from build123d import *

# Parameters (mm, degrees)
BOSS_EXTRUDE1_DEPTH   = 1.6
F_4_0MM_DOWEL_HOLE1_D = 4


with BuildPart() as part:
    # Sketch1 → Boss-Extrude1 (new body)
    with BuildSketch(Plane(origin=(0, 0, 0), x_dir=(1, 0, 0), z_dir=(0, 1, 0))):
        with BuildLine():
            ThreePointArc((-65, 33.226495452), (-73, 0), (-65, -33.226495452))
            ThreePointArc((-65, -33.226495452), (-51.618795027, -51.618795027), (-33.226495452, -65))
            ThreePointArc((-33.226495452, -65), (0, -73), (33.226495452, -65))
            ThreePointArc((33.226495452, -65), (51.618795027, -51.618795027), (65, -33.226495452))
            ThreePointArc((65, -33.226495452), (70.971825396, -17.088007491), (73, 0))
            ThreePointArc((73, 0), (70.971825396, 17.088007491), (65, 33.226495452))
            ThreePointArc((65, 33.226495452), (51.618795027, 51.618795027), (33.226495452, 65))
            ThreePointArc((33.226495452, 65), (0, 73), (-33.226495452, 65))
            ThreePointArc((-33.226495452, 65), (-51.618795027, 51.618795027), (-65, 33.226495452))
        make_face()
    extrude(amount=BOSS_EXTRUDE1_DEPTH)

    # Ø4.0mm Dowel Hole1 (through all)
    with Locations(Plane(origin=(0, 1.6, 0), x_dir=(1, 0, 0), z_dir=(0, 1, 0))):
        with Locations((0, 55), (55, 0), (-55, 0), (0, -55)):
            Hole(F_4_0MM_DOWEL_HOLE1_D / 2)


solid = part.part
Could you check a few things on this model? Use its own coordinates, in mm. Coordinates: 2 decimals unless noted, no trailing zeros. Order: outer loops, then holes, each group sorted by start corner. A loop starts at its lowest first (then second) coordinate and runs counter-clockwise, first axis right, second up. Notation, with made-up numbers: (46, -6) -> (86, -6) arc R23 cw to (86, 28) -> close; hole circle Ø6 at (-26.5, 38). An arc over 180 degrees is marked (long way). One line per item, written item: value. Start each with the question number.
1) Imagine slicing it at D-D on y = 0.8. List the corners of the cut face in (x, z) for me.
2) Imagine slicing it at A-A on x = 0. List the corners of the cut face in (y, z) for me.
3) Imagine slicing it at C-C on x = -55. List the corners of the cut face in (y, z) for me.
4) Imagine slicing it at B-B on z = 55. List the corners of the cut face in (x, y) for me, plus the area to 3 significant figures.
5) We'd pull the mould along X, two halves only. Please class faces 1 (the cylindrical face through (0, 1, 53)), 2 (the flat face through (-1, 0, -1)): +X half, -X half, draft (parallel to the pull), parting line (faces both ways), or undercut.
6) If I drill on L1, parallel to Z at x = 55, y = 0.6; L2, parallel to X at y = 0.3, z = -34.5, over which ranges is the centre line in solid material (lowest first)? Write a range as [from, to].
Answer list:
1. outline: circle Ø146 at (0, 0); hole circle Ø4 at (-55, 0); hole circle Ø4 at (0, -55); hole circle Ø4 at (0, 55); hole circle Ø4 at (55, 0)
2. outline: (0, -73) -> (1.6, -73) -> (1.6, -57) -> (0, -57) -> close; (0, -53) -> (1.6, -53) -> (1.6, 53) -> (0, 53) -> close; (0, 57) -> (1.6, 57) -> (1.6, 73) -> (0, 73) -> close
3. outline: (0, -48) -> (1.6, -48) -> (1.6, -2) -> (0, -2) -> close; (0, 2) -> (1.6, 2) -> (1.6, 48) -> (0, 48) -> close
4. outline: (-48, 0) -> (-2, 0) -> (-2, 1.6) -> (-48, 1.6) -> close; (2, 0) -> (48, 0) -> (48, 1.6) -> (2, 1.6) -> close
4. area: 147 mm2
5. face 1: undercut
5. face 2: draft
6. L1: z = [-48, -2], [2, 48]
6. L2: x = [-64.33, 64.33]
